from build123d import *

# Parameters (mm, degrees)
SKETCH1_W                  = 90
SKETCH1_H                  = 82
BOSS_EXTRUDE1_DEPTH        = 6
M8_CLEARANCE_HOLE1_D       = 8.4
CUT_EXTRUDE1_DEPTH         = 94.728330829
CUT_EXTRUDE1_DEPTH_BACK    = 12
SKETCH6_W                  = 35
SKETCH6_H                  = 12
F_12_0_12_DIAMETER_HOLE1_D = 12
M6_TAPPED_HOLE1_D          = 5
M6_TAPPED_HOLE1_DEPTH      = 15.497848452
M6_TAPPED_HOLE1_TIP        = 1.502151548


with BuildPart() as part:
    # Sketch1 → Boss-Extrude1 (new, symmetric)
    with BuildSketch(Plane.XY):
        Rectangle(SKETCH1_W, SKETCH1_H)
    extrude(amount=BOSS_EXTRUDE1_DEPTH, both=True)

    # M8 Clearance Hole1 (through all)
    with Locations(Plane.XY.offset(6)):
        with Locations((-35, 17), (35, 17), (35, -29), (-35, -29), (-35, 35), (35, 35)):
            Hole(M8_CLEARANCE_HOLE1_D / 2)

    # Sketch6 → Cut-Extrude1 (cut, two sides: drawn at the far end of the back side and taken through both)
    with BuildSketch(Plane(origin=(0, 41, 0), x_dir=(1, 0, 0), z_dir=(0, 1, 0)).offset(-CUT_EXTRUDE1_DEPTH_BACK)):
        Rectangle(SKETCH6_W, SKETCH6_H)
    extrude(amount=CUT_EXTRUDE1_DEPTH + CUT_EXTRUDE1_DEPTH_BACK, mode=Mode.SUBTRACT)

    # Ø12.0 (12) Diameter Hole1 (through all)
    with Locations(Plane.XY.offset(6)):
        with Locations((0, -1)):
            Hole(F_12_0_12_DIAMETER_HOLE1_D / 2)

    # M6 Tapped Hole1
    with Locations(Plane(origin=(0, 29, 0), x_dir=(1, 0, 0), z_dir=(0, 1, 0))):
        with Locations((-7.5, 0), (7.5, 0)):
            Hole(M6_TAPPED_HOLE1_D / 2, depth=M6_TAPPED_HOLE1_DEPTH)
            with Locations((0, 0, -(M6_TAPPED_HOLE1_DEPTH + M6_TAPPED_HOLE1_TIP / 2))):  # 118° drill point
                Cone(0, M6_TAPPED_HOLE1_D / 2, M6_TAPPED_HOLE1_TIP, mode=Mode.SUBTRACT)


solid = part.part
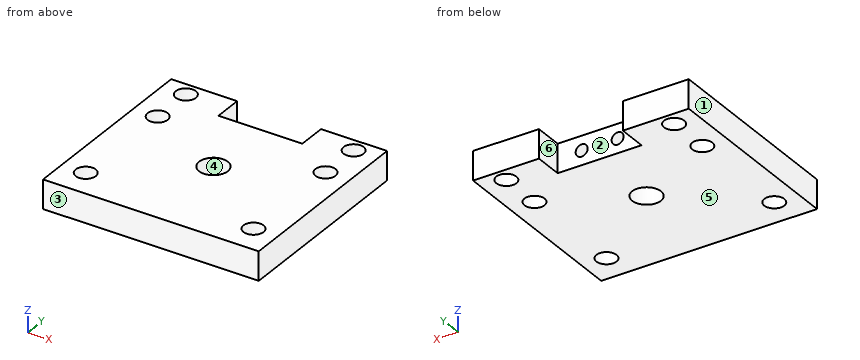
Work out the finished part from the listing and answer in its coordinate system (mm). Face numbers are marked on the shaded views. A direction names the side the tool comes from. Give positions to 0.01 mm unless a question says otherwise; leave off trailing zeros. Order: outer loops, then holes, each group sorted by start corner. A loop starts at its lowest first (then second) coordinate and runs counter-clockwise, first axis right, second up. Notation, with made-up numbers: M 75,-37.5 L 101,-37.5 A16 ccw 101,-12.5 Z; hole C 36,31.5 d11. An arc over 180 degrees is marked long. Return JSON: item names as keys, results as strings.
Q1. Which of the six approach directions +Z, -Z, +X, -X, +Y, -Y give full straight-line access (tool end or side, diameter ignored) to the marked faces 5 and 6?
Answer below:
{"face 5": "-Z, +X, -X, +Y, -Y", "face 6": "+Z, -Z, +Y"}
Q2. Find section A-A, the plane y = 17. Write down the section's boundary in (x, z).
Answer below:
{"outline": "M -45,-6 L -39.2,-6 L -39.2,6 L -45,6 Z; M -30.8,-6 L 30.8,-6 L 30.8,6 L -30.8,6 Z; M 39.2,-6 L 45,-6 L 45,6 L 39.2,6 Z; hole C -7.5,0 d5; hole C 7.5,0 d5"}
Q3. Find section C-C, the plane z = 3.5. Write down the section's boundary in (x, y).
Answer below:
{"outline": "M -45,-41 L 45,-41 L 45,41 L 17.5,41 L 17.5,29 L -17.5,29 L -17.5,41 L -45,41 Z; hole C -35,-29 d8.4; hole C -35,17 d8.4; hole C -35,35 d8.4; hole C 0,-1 d12; hole C 35,-29 d8.4; hole C 35,17 d8.4; hole C 35,35 d8.4"}
Q4. Find the intervals of material crossed by line 1 along Y through (x, z) = (-35, 1.75); line 2 along X through (y, z) = (30, 3.25); line 3 along X through (y, z) = (32.5, -4.75), in increasing order. Write a range as [from, to].
Answer below:
{"line 1": "y = [-41, -33.2], [-24.8, 12.8], [21.2, 30.8], [39.2, 41]", "line 2": "x = [-45, -17.5], [17.5, 45]", "line 3": "x = [-45, -38.37], [-31.63, -17.5], [17.5, 31.63], [38.37, 45]"}
Q5. This flat-tipped pin is pushed along its axis until it touches: pin 1 (7.5 mm diameter, centred on x = -35, y = 17, fed in from +Z). Where does it stop, or does it pass through?
Answer below:
{"pin 1": "passes through"}
Q6. The mould has two halves that part along X. Classify the marked faces 1, 2, 3 and 4: pulls with the +X half, pulls with the -X half, needs draft (parallel to the pull), parting line crosses it, or undercut.
Answer below:
{"face 1": "pulls with the -X half", "face 2": "undercut", "face 3": "needs draft", "face 4": "undercut"}
Q7. Find section B-B, the plane x = -35. Write down the section's boundary in (y, z).
Answer below:
{"outline": "M -41,-6 L -33.2,-6 L -33.2,6 L -41,6 Z; M -24.8,-6 L 12.8,-6 L 12.8,6 L -24.8,6 Z; M 21.2,-6 L 30.8,-6 L 30.8,6 L 21.2,6 Z; M 39.2,-6 L 41,-6 L 41,6 L 39.2,6 Z"}
Q8. Find section D-D, the plane x = 0. Write down the section's boundary in (y, z), and give its area (3 significant figures).
Answer below:
{"outline": "M -41,-6 L -7,-6 L -7,6 L -41,6 Z; M 5,-6 L 29,-6 L 29,6 L 5,6 Z", "area": "696 mm^2"}
